Read the model definition and answer for the solid it produces. Units are mm, in the model's axes. A direction names the side the tool comes from. Coordinates: 2 decimals unless noted, no trailing zeros. Loops run counter-clockwise (first coordinate to the right, second up) from the corner with the lowest first, then second, coordinate; pieces in that order, holes last. Notation, with made-up numbers: (11.5, 21.25) -> (54.5, 21.25) arc R17 cw to (54.5, 33.25) -> close; hole circle Ø1 at (9.25, -1.75). An arc over 180 degrees is marked (long way). Answer as CSV lines item,"result".
```python
from build123d import *

# Parameters (mm, degrees)
SKETCH_1_R               = 38.598396019
EXTRUDE_1_DEPTH          = 4.4
SKETCH_2_R               = 36.869922329
SKETCH_2_R_2             = 34.869922329
CUT_EXTRUDE_1_DEPTH      = 0.6
SKETCH_3_W               = 5
SKETCH_3_H               = 9
EXTRUDE_2_DEPTH          = 14.5
FILLET_2_R               = 4.5
CUT_EXTRUDE_2_DEPTH      = 59.216529702
CUT_EXTRUDE_2_DEPTH_BACK = 59.216529702
SKETCH_4_R               = 1.55
CUT_EXTRUDE_3_DEPTH      = 57.479397575
CUT_EXTRUDE_3_DEPTH_BACK = 57.479397575
SKETCH_5_R               = 1.25


with BuildPart() as part:
    # 스케치1 → 보스-돌출1 (new body)
    with BuildSketch(Plane(origin=(0, 0, 0), x_dir=(1, 0, 0), z_dir=(0, 1, 0))):
        with Locations(Location((0, 0, 0), (0, 0, 270))):
            Circle(SKETCH_1_R)
    extrude(amount=EXTRUDE_1_DEPTH)

    # 스케치2 → 컷-돌출1 (cut)
    with BuildSketch(Plane(origin=(0, 4.4, 0), x_dir=(1, 0, 0), z_dir=(0, 1, 0))):
        with Locations(Location((0, 0, 0), (0, 0, 270))):
            Circle(SKETCH_2_R)
        with Locations(Location((0, 0, 0), (0, 0, 270))):
            Circle(SKETCH_2_R_2, mode=Mode.SUBTRACT)
    extrude(amount=-CUT_EXTRUDE_1_DEPTH, mode=Mode.SUBTRACT)

    # 스케치3 → 보스-돌출2 (add)
    with BuildSketch(Plane.XZ):
        with Locations((0, -15)):
            Rectangle(SKETCH_3_W, SKETCH_3_H)
        with Locations((0, 15)):
            Rectangle(SKETCH_3_W, SKETCH_3_H)
    extrude(amount=EXTRUDE_2_DEPTH)

    # 필렛2
    fillet_2_edges = [part.edges().sort_by_distance(p)[0] for p in [
        (0, -14.5, -19.5),
        (0, -14.5, -10.5),
        (0, -14.5, 19.5),
        (0, -14.5, 10.5),
    ]]
    fillet(fillet_2_edges, radius=FILLET_2_R - 0.0001)  # a hair under: the kernel refuses the full size

    # 스케치4 → 컷-돌출2 (cut, two sides: drawn at the far end of the back side and taken through both)
    with BuildSketch(Plane.ZY.offset(2.5).offset(-CUT_EXTRUDE_2_DEPTH_BACK)):
        with Locations((-15, -10)):
            Circle(SKETCH_4_R)
        with Locations((15, -10)):
            Circle(SKETCH_4_R)
    extrude(amount=CUT_EXTRUDE_2_DEPTH + CUT_EXTRUDE_2_DEPTH_BACK, mode=Mode.SUBTRACT)

    # 스케치5 → 컷-돌출3 (cut, two sides: drawn at the far end of the back side and taken through both)
    with BuildSketch(Plane.XZ.offset(-CUT_EXTRUDE_3_DEPTH_BACK)):
        with Locations(Location((17.7, 0, 0), (0, 0, 270))):
            Circle(SKETCH_5_R)
    extrude(amount=CUT_EXTRUDE_3_DEPTH + CUT_EXTRUDE_3_DEPTH_BACK, mode=Mode.SUBTRACT)


solid = part.part
```
Q1. A cutting plane is placed at B-B, the plane z = 0. Write down the section's boundary in (x, y).
Results:
outline,"(-38.6, 0) -> (16.45, 0) -> (16.45, 4.4) -> (-34.87, 4.4) -> (-34.87, 3.8) -> (-36.87, 3.8) -> (-36.87, 4.4) -> (-38.6, 4.4) -> close; (18.95, 0) -> (38.6, 0) -> (38.6, 4.4) -> (36.87, 4.4) -> (36.87, 3.8) -> (34.87, 3.8) -> (34.87, 4.4) -> (18.95, 4.4) -> close"
Q2. A cutting plane is placed at C-C, the plane x = 0. Give the number of separate pieces and of enclosed holes in the cut face, and give its area (3 significant figures).
Results:
separate pieces,"1"
enclosed holes,"2"
area,"566 mm²"
Q3. Find the intervals of material crossed by probe 1 along Z at (x, y) = (-0.4, -10); probe 2 along X at (y, z) = (4, 0); probe 3 along Z at (x, y) = (0.5, -5.5), in increasing order. Write a range as [from, to].
Results:
probe 1,"z = [-19.5, -16.55], [-13.45, -10.5], [10.5, 13.45], [16.55, 19.5]"
probe 2,"x = [-38.6, -36.87], [-34.87, 16.45], [18.95, 34.87], [36.87, 38.6]"
probe 3,"z = [-19.5, -10.5], [10.5, 19.5]"
Q4. For faces 5 (the face through (0.035, -13.147, -11.783)), 6 (the face through (0, -5, -19.5)), 7 (the face through (0, -5, 19.5)), determine the directions among +Z, -Z, +X, -X, +Y, -Y from which every point of the face is accessible in a straight line to the end or side of a thin tool.
Results:
face 5,"+X, -X, -Y"
face 6,"-Z, +X, -X, -Y"
face 7,"+Z, +X, -X, -Y"
Q5. A cutting plane is placed at A-A, the plane y = -1. Write down the section's boundary in (x, z).
Results:
outline,"(-2.5, -19.5) -> (2.5, -19.5) -> (2.5, -10.5) -> (-2.5, -10.5) -> close; (-2.5, 10.5) -> (2.5, 10.5) -> (2.5, 19.5) -> (-2.5, 19.5) -> close"
Q6. Given pin 1 Ø4 at (y, z) = (-10, 15) entering from -X; pin 2 Ø1.5 at (x, y) = (0, -7.5) entering from +Z; pin 3 Ø6 at (x, y) = (-6, -1.5) entering from +Z, each flat-ended and moving along its own axis, determine where each tip first touches the part or whether it passes through.
Results:
pin 1,"stops at x = -2.5"
pin 2,"stops at z = 19.5"
pin 3,"stops at z = 38.45"
Q7. A cutting plane is placed at D-D, the plane x = 17.7. Write down the section's boundary in (y, z), and give its area (3 significant figures).
Results:
outline,"(0, -34.3) -> (4.4, -34.3) -> (4.4, -32.34) -> (3.8, -32.34) -> (3.8, -30.04) -> (4.4, -30.04) -> (4.4, -1.25) -> (0, -1.25) -> close; (0, 1.25) -> (4.4, 1.25) -> (4.4, 30.04) -> (3.8, 30.04) -> (3.8, 32.34) -> (4.4, 32.34) -> (4.4, 34.3) -> (0, 34.3) -> close"
area,"288 mm²"
Q8. For a pull along X with two mould halves and no side action, classify faces 1 (the face through (0.03, -9.93, -16.55)), 2 (the face through (2.5, -7, 15)), 3 (the face through (-23.49, 2.17, -30.63)), 4 (the face through (-21.22, 4.1, -27.67)) as pulls with the +X half, pulls with the -X half, needs draft (parallel to the pull), parting line crosses it, or undercut.
Results:
face 1,"needs draft"
face 2,"pulls with the +X half"
face 3,"parting line crosses it"
face 4,"undercut"
